Here's how the part is built. I have some questions about the finished solid (model axes, mm). Face numbers are marked on the shaded views. A direction names the side the tool comes from. Coordinates: 2 decimals unless noted, no trailing zeros. Write each loop counter-clockwise with the first axis right and the second up, starting at its lowest first coordinate (ties: lowest second). Pieces come first, ordered by that corner, then holes.
Autodesk Inventor part; units mm, degrees
ref_plane "YZ Plane" through (0, 0, 0) normal (1, 0, 0) x (0, 1, 0)
ref_plane "XZ Plane" through (0, 0, 0) normal (0, 1, 0) x (-1, 0, 0)
ref_plane "XY Plane" through (0, 0, 0) normal (0, 0, 1) x (1, 0, 0)
sketch "Náčrt1" plane through (0, 0, 0) normal (0, 1, 0) x (-1, 0, 0)
  circle A0 centre (0, 0) radius 3.1
  circle A1 centre (0, 0) radius 1.45
  line L0 (3.1, 0) -> (-3.1, 0)
  line L1 (-3.1, 0) -> (-3.1, 3.1)
  line L2 (-3.1, 3.1) -> (3.1, 3.1)
  line L3 (3.1, 3.1) -> (3.1, 0)
  point P0 (0, 3.1)
  dimension "d0" = 6.2
  dimension "d1" = 2.9
extrude "Vysunutí1" add sketch "Náčrt1" against normal blind 42 contours L0 A1 A0 | A0 L0 A1 | L0 A1 | A1 L0
extrude "Vysunutí2" add sketch "Náčrt1" against normal blind 27 contours L1 L2 A0 | A0 L2 L3
sketch "Náčrt2" plane through (0, 0, 0) normal (0, 1, 0) x (1, 0, 0)
  circle A0 centre (0, 0) radius 3.1
  point P0 (-3.1, 0)
  point P1 (3.1, 0)
hole "Díra1" at (0, 0, 0) direction (0, -1, 0) diameter 2.9 depth 10
sketch "Náčrt3" plane through (0, -42, 0) normal (0, -1, 0) x (1, 0, 0)
  circle A0 centre (0, 0) radius 3.1
  point P0 (3.1, 0)
  point P1 (-3.1, 0)
hole "Díra2" at (0, -42, 0) direction (0, 1, 0) diameter 2.85 depth 4.5
properties part number "spojka v2"
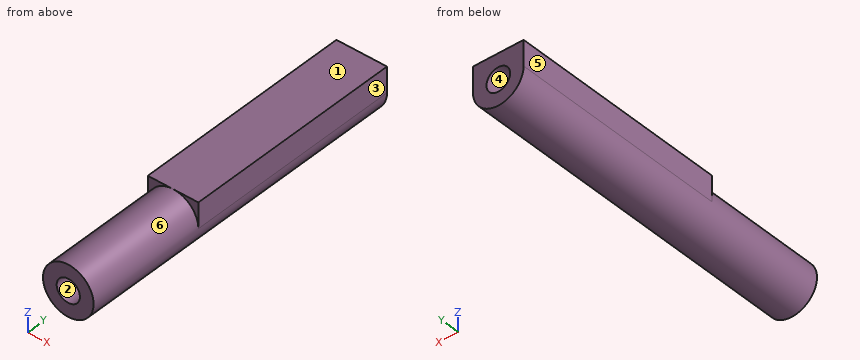
1. Thinking about a two-plate mould opening in Z: for the marked faces 1, 2, 3 and 4, which applies, pulls with the +Z half, pulls with the -Z half, needs draft (parallel to the pull), parting line crosses it, or undercut?
2. I want a section at C-C (z = -1). List the corners of the cut face in (x, y) for me, then the cut area to 3 significant figures.
3. For pin 1 Ø1 at (x, y) = (-1, -34) entering from +Z, with a flat end and sliding along its axis, tell me the tip position at first contact or that it passes through.
4. I want a section at B-B (x = -2). List the corners of the cut face in (y, z) for me.
5. I want a section at A-A (y = -6.5). List the corners of the cut face in (x, z) for me, then the cut area to 3 significant figures.
6. On a 3-axis mill with a long thin cutter (end or side, diameter ignored), from which of +Z, -Z, +X, -X, +Y, -Y can I reach the whole of each face in a straight line? I mean the marked faces 5 and 6. Say none if no direction works.
7. If I drill on line 1 (Z direction, x = 0, y = -38.75) (3 decimals); line 2 (X direction, y = -7, z = 0); line 3 (Y direction, x = 0.5, z = -1), over which ranges is the centre line in solid material (lowest first)?
8. I want a section at D-D (y = -18.5). List the corners of the cut face in (x, z) for me, then the cut area to 3 significant figures.
Response values:
1. face 1: pulls with the +Z half
1. face 2: undercut
1. face 3: needs draft
1. face 4: undercut
2. outline: (-2.93, -42) - (-1.02, -42) - (-1.02, -37.5) - (1.02, -37.5) - (1.02, -42) - (2.93, -42) - (2.93, 0) - (1.05, 0) - (1.05, -10) - (-1.05, -10) - (-1.05, 0) - (-2.93, 0) - close
2. area: 216 mm2
3. pin 1: stops at z = 3.06
4. outline: (-42, -2.37) - (0, -2.37) - (0, 3.1) - (-27, 3.1) - (-27, 2.37) - (-42, 2.37) - close
5. outline: (-3.1, 0) arc R3.1 ccw to (3.1, 0) - (3.1, 3.1) - (-3.1, 3.1) - close; hole circle Ø2.9 at (0, 0)
5. area: 27.7 mm2
6. face 5: +Z, -Z, -X, +Y, -Y
6. face 6: -Y
7. line 1: z = -3.1 to -1.425, 1.425 to 3.1
7. line 2: x = -3.1 to -1.45, 1.45 to 3.1
7. line 3: y = -37.5 to -10
8. outline: (-3.1, 0) arc R3.1 ccw to (3.1, 0) - (3.1, 3.1) - (-3.1, 3.1) - close
8. area: 34.3 mm2
